Geometry check sheet. Reference: the model listing, model coordinates, mm. Round coordinates to 2 decimals unless told otherwise and drop trailing zeros. Loops run counter-clockwise (first coordinate to the right, second up) from the corner with the lowest first, then second, coordinate; pieces in that order, holes last. Notation, with made-up numbers: (37.5, -26) -> (43.5, -26) arc R26 ccw to (43.5, 2) -> close; hole circle Ø1 at (31.25, 58). An arc over 180 degrees is marked (long way). Use a Markdown table: item, result. Add a question column.
Q1. Material ranges on L1, parallel to X at y = -102, z = 1.8; L2, parallel to X at y = -445, z = 1.8; L3, parallel to X at y = -332.18, z = 1, recorded low to high.
Q2. Sectioned sample at B-B, the plane y = -107. Enter the section's corners in (x, z).
Q3. Gauge pin test, flat ends, axial feed: P1, Ø1.5, axis at x = 53.5, z = 1.5, coming from the +Y side; P2, Ø1.5, axis at y = -473, z = 1, coming from the +X side; P3, Ø0.9, axis at y = -366.5, z = 2, coming from the -X side; P4, Ø6, axis at x = 35.5, y = -116, coming from the -Z side. Record the tip position at first contact, or that the pin passes through.
Q4. Sectioned sample at A-A, the plane y = -43.5. Enter the section's corners in (x, z), then the cut area to 3 significant figures.
Q5. Sectioned sample at C-C, the plane z = 1.8. Give the number of separate pieces and of enclosed holes in the cut face, then the cut area to 3 significant figures.
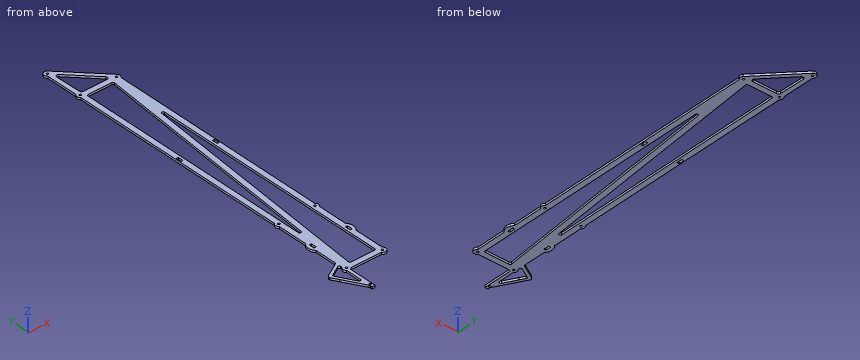
```python
from build123d import *

# Parameters (mm, degrees)
SKETCH_1_R      = 1.5
SKETCH_1_W      = 3.04
SKETCH_1_H      = 8.04
EXTRUDE_1_DEPTH = 3


with BuildPart() as part:
    # 草图1 → 凸台-拉伸1 (new body)
    with BuildSketch(Plane.XY):
        with BuildLine():
            Line((-3, -4), (-3, -328.18))
            ThreePointArc((-3, -328.18), (-5, -332.18), (-3, -336.18))
            Line((-3, -336.18), (-3, -379.66982063))
            ThreePointArc((-3, -379.66982063), (-6.694859274, -388.59), (-3, -397.51017937))
            Line((-3, -397.51017937), (-3, -429.017949192))
            ThreePointArc((-3, -429.017949192), (-3.401923789, -430.517949192), (-4.5, -431.616025404))
            Line((-4.5, -431.616025404), (-25.083647797, -443.5))
            ThreePointArc((-25.083647797, -443.5), (-26.481425275, -445.321619076), (-26.181724008, -447.598076211))
            Line((-26.181724008, -447.598076211), (-20.646282865, -457.185741513))
            Line((-20.646282865, -457.185741513), (-3.401923789, -487.053847577))
            ThreePointArc((-3.401923789, -487.053847577), (-3.102222521, -487.777390442), (-3, -488.553847577))
            Line((-3, -488.553847577), (-3, -491.25))
            Line((-3, -491.25), (1.5, -491.25))
            Line((1.5, -491.25), (1.5, -487.35037357))
            Line((1.5, -487.35037357), (1.5, -485.14962643))
            Line((1.5, -485.14962643), (1.5, -449.769696007))
            ThreePointArc((1.5, -449.769696007), (2.888850289, -449.080997918), (4, -448))
            Line((4, -448), (49, -448))
            ThreePointArc((49, -448), (56.535533906, -448.535533906), (56, -441))
            Line((56, -441), (56, -397.51017937))
            ThreePointArc((56, -397.51017937), (59.694859274, -388.59), (56, -379.66982063))
            Line((56, -379.66982063), (56, -336.18))
            ThreePointArc((56, -336.18), (58, -332.18), (56, -328.18))
            Line((56, -328.18), (56, -4))
            ThreePointArc((56, -4), (57.987421044, -0.3544451), (56.535533906, 3.535533906))
            Line((56.535533906, 3.535533906), (3, 59))
            ThreePointArc((3, 59), (-4, 58), (-3, 51))
            Line((-3, 51), (-3, 4))
            ThreePointArc((-3, 4), (-5, 0), (-3, -4))
        make_face()
        Circle(SKETCH_1_R, mode=Mode.SUBTRACT)
        with Locations((0, -445)):
            Circle(SKETCH_1_R, mode=Mode.SUBTRACT)
        with Locations((0, -332.18)):
            Circle(SKETCH_1_R, mode=Mode.SUBTRACT)
        with Locations(Location((53, -332.18, 0), (0, 0, 180))):
            Circle(SKETCH_1_R, mode=Mode.SUBTRACT)
        with Locations(Location((53, -445, 0), (0, 0, 180))):
            Circle(SKETCH_1_R, mode=Mode.SUBTRACT)
        with Locations(Location((53, 0, 0), (0, 0, 180))):
            Circle(SKETCH_1_R, mode=Mode.SUBTRACT)
        with Locations((0, 55)):
            Circle(SKETCH_1_R, mode=Mode.SUBTRACT)
        with Locations((-1, -486.25)):
            Circle(SKETCH_1_R, mode=Mode.SUBTRACT)
        with BuildLine():
            Line((6.938150971, 3), (41.969807465, 3))
            ThreePointArc((41.969807465, 3), (44.729078046, 4.822534134), (44.135772081, 8.07571609))
            Line((44.135772081, 8.07571609), (8.325634331, 45.44281635))
            ThreePointArc((8.325634331, 45.44281635), (5.012233456, 46.138993121), (3.160320545, 43.30461382))
            Line((3.160320545, 43.30461382), (3.938801801, 5.937513559))
            ThreePointArc((3.938801801, 5.937513559), (4.839039174, 3.85670122), (6.938150971, 3))
        make_face(mode=Mode.SUBTRACT)
        with BuildLine():
            Line((48, -86.226063366), (48, -438))
            ThreePointArc((48, -438), (47.414213562, -439.414213562), (46, -440))
            Line((46, -440), (11.226944195, -440))
            ThreePointArc((11.226944195, -440), (9.744803089, -439.342854326), (9.236644598, -437.803257741))
            Line((9.236644598, -437.803257741), (44.009700404, -86.029321107))
            ThreePointArc((44.009700404, -86.029321107), (46.098490627, -84.228489939), (48, -86.226063366))
        make_face(mode=Mode.SUBTRACT)
        with BuildLine():
            Line((43.763355402, -7.196742259), (8.990299596, -358.970678893))
            ThreePointArc((8.990299596, -358.970678893), (6.901509373, -360.771510061), (5, -358.773936634))
            Line((5, -358.773936634), (5, -7))
            ThreePointArc((5, -7), (5.585786438, -5.585786438), (7, -5))
            Line((7, -5), (41.773055805, -5))
            ThreePointArc((41.773055805, -5), (43.255196911, -5.657145674), (43.763355402, -7.196742259))
        make_face(mode=Mode.SUBTRACT)
        with BuildLine():
            Line((-17.18218125, -455.185741513), (-21.217622393, -448.196152423))
            ThreePointArc((-21.217622393, -448.196152423), (-21.417423238, -446.678514333), (-20.485571585, -445.464101615))
            Line((-20.485571585, -445.464101615), (-6, -437.100852961))
            ThreePointArc((-6, -437.100852961), (-4, -437.100852961), (-3, -438.832903769))
            Line((-3, -438.832903769), (-3, -441))
            ThreePointArc((-3, -441), (-5, -445), (-3, -449))
            Line((-3, -449), (-3, -472.285898385))
            ThreePointArc((-3, -472.285898385), (-4.48236191, -474.217750037), (-6.732050808, -473.285898385))
            Line((-6.732050808, -473.285898385), (-17.18218125, -455.185741513))
        make_face(mode=Mode.SUBTRACT)
        Polygon((-1.52, -388.59), (-1.52, -384.57), (1.52, -384.57), (1.52, -392.61), (-1.52, -392.61), align=None, mode=Mode.SUBTRACT)
        Polygon((54.52, -392.61), (54.52, -388.59), (54.52, -384.57), (51.48, -384.57), (51.48, -392.61), align=None, mode=Mode.SUBTRACT)
        with Locations((53, -166.09)):
            Rectangle(SKETCH_1_W, SKETCH_1_H, mode=Mode.SUBTRACT)
        with Locations((0, -166.09)):
            Rectangle(SKETCH_1_W, SKETCH_1_H, mode=Mode.SUBTRACT)
    extrude(amount=EXTRUDE_1_DEPTH)


solid = part.part
```
Values:
| question | item | result |
|---|---|---|
| 1 | L1 | -3 to 5, 34.39 to 42.43, 48 to 56 |
| 1 | L2 | -26.38 to -19.68, -5 to -1.5, 1.5 to 51.5, 54.5 to 58 |
| 1 | L3 | -5 to -1.5, 1.5 to 5, 11.64 to 19.68, 48 to 51.5, 54.5 to 58 |
| 2 | outline | (-3, 0) -> (5, 0) -> (5, 3) -> (-3, 3) -> close; (33.9, 0) -> (41.94, 0) -> (41.94, 3) -> (33.9, 3) -> close; (48, 0) -> (56, 0) -> (56, 3) -> (48, 3) -> close |
| 3 | P1 | y = 7.46 |
| 3 | P2 | x = 1.5 |
| 3 | P3 | x = -3 |
| 3 | P4 | z = 0 |
| 4 | outline | (-3, 0) -> (5, 0) -> (5, 3) -> (-3, 3) -> close; (40.17, 0) -> (56, 0) -> (56, 3) -> (40.17, 3) -> close |
| 4 | area | 71.5 mm^2 |
| 5 | separate pieces | 1 |
| 5 | enclosed holes | 16 |
| 5 | area | 12,700 mm^2 |
